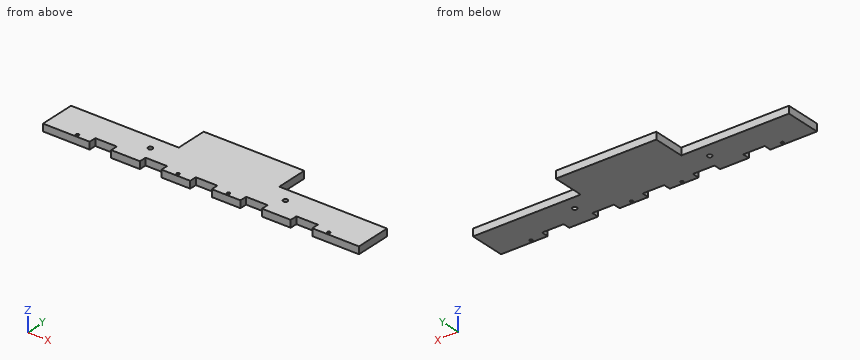
```python
from build123d import *

# Parameters (mm, degrees)
SKETCH_1_W          = 220
SKETCH_1_H          = 25
EXTRUDE_1_DEPTH     = 5
SKETCH_2_W          = 70
SKETCH_2_H          = 22.26349322
EXTRUDE_2_DEPTH     = 5
SKETCH_3_W          = 15
SKETCH_3_H          = 5
CUT_EXTRUDE_1_DEPTH = 226.075182531
SKETCH_4_R          = 1.6
CUT_EXTRUDE_2_DEPTH = 226.075182531
SKETCH_7_R          = 1
CUT_EXTRUDE_4_DEPTH = 226.075182531


with BuildPart() as part:
    # 草图1 → 凸台-拉伸1 (new body)
    with BuildSketch(Plane.XY):
        with Locations((110, 12.5)):
            Rectangle(SKETCH_1_W, SKETCH_1_H)
    extrude(amount=EXTRUDE_1_DEPTH)

    # 草图2 → 凸台-拉伸2 (add)
    with BuildSketch(Plane.XY.offset(5)):
        with Locations((110, 36.13174661)):
            Rectangle(SKETCH_2_W, SKETCH_2_H)
    extrude(amount=-EXTRUDE_2_DEPTH)

    # 草图3 → 切除-拉伸1 (cut, through all)
    with BuildSketch(Plane.XY.offset(5)):
        with Locations((110, 2.5)):
            Rectangle(SKETCH_3_W, SKETCH_3_H)
        with Locations((145, 2.5)):
            Rectangle(SKETCH_3_W, SKETCH_3_H)
        with Locations((180, 2.5)):
            Rectangle(SKETCH_3_W, SKETCH_3_H)
        with Locations((75, 2.5)):
            Rectangle(SKETCH_3_W, SKETCH_3_H)
        with Locations((40, 2.5)):
            Rectangle(SKETCH_3_W, SKETCH_3_H)
    extrude(amount=-CUT_EXTRUDE_1_DEPTH, mode=Mode.SUBTRACT)

    # 草图4 → 切除-拉伸2 (cut, through all)
    with BuildSketch(Plane.XY.offset(5)):
        with Locations((63, 15)):
            Circle(SKETCH_4_R)
        with Locations((157, 15)):
            Circle(SKETCH_4_R)
    extrude(amount=-CUT_EXTRUDE_2_DEPTH, mode=Mode.SUBTRACT)

    # 草图7 → 切除-拉伸4 (cut, through all)
    with BuildSketch(Plane.XY.offset(5)):
        with Locations((22.5, 2)):
            Circle(SKETCH_7_R)
        with Locations((92.5, 2)):
            Circle(SKETCH_7_R)
        with Locations((127.5, 2)):
            Circle(SKETCH_7_R)
        with Locations((197.5, 2)):
            Circle(SKETCH_7_R)
    extrude(amount=-CUT_EXTRUDE_4_DEPTH, mode=Mode.SUBTRACT)


solid = part.part
```
Can you work these out from the model? Positions are in its coordinate system, mm. Coordinates: 2 decimals unless noted, no trailing zeros. Loops run counter-clockwise (first coordinate to the right, second up) from the corner with the lowest first, then second, coordinate; pieces in that order, holes last. Notation, with made-up numbers: M -10.5,4.5 L 2.5,4.5 A5 cw 2.5,13.5 Z; hole C 37,37.5 d10. An arc over 180 degrees is marked long. Put each result on its own line as item: value. Start each with the question number.
(1) I need wall thicknesses on probe 1 along Y at (x, z) = (127.5, 2.05); probe 2 along Y at (x, z) = (157, 3.9); probe 3 along X at (y, z) = (41, 1.8). Which ranges of each line are inside material? Lowest first, please.
(2) Imagine slicing it at A-A on z = 2. Give the number of separate pieces and of enclosed holes in the cut face, and give its area (3 significant figures).
(3) Will these pins go through, and if not, where does the flat tip stop? pin 1 Ø1 at (x, z) = (64.5, 2.5) entering from +Y; pin 2 Ø2 at (y, z) = (36.5, 1) entering from -X.
(4) Imagine slicing it at B-B on x = 162. List the corners of the cut face in (y, z) for me, and give its area (3 significant figures).
(5) Imagine slicing it at C-C on y = 40. List the corners of the cut face in (x, z) for me.
Worked answers:
1. probe 1: y = 0 to 1, 3 to 47.26
1. probe 2: y = 0 to 13.4, 16.6 to 25
1. probe 3: x = 75 to 145
2. separate pieces: 1
2. enclosed holes: 6
2. area: 6,650 mm2
3. pin 1: stops at y = 25
3. pin 2: stops at x = 75
4. outline: M 0,0 L 25,0 L 25,5 L 0,5 Z
4. area: 125 mm2
5. outline: M 75,0 L 145,0 L 145,5 L 75,5 Z
